Design review of the part built by this model. Coordinates are the model's own, in mm. A direction names the side the tool comes from. Give positions to 0.01 mm unless a question says otherwise; leave off trailing zeros. Write each loop counter-clockwise with the first axis right and the second up, starting at its lowest first coordinate (ties: lowest second). Pieces come first, ordered by that corner, then holes. Notation, with made-up numbers: M 42.25,86 L 90.25,86 A35 ccw 90.25,124 Z; hole C -23,48.5 d10. An arc over 180 degrees is marked long. Answer in a Markdown table with one row per item.
```python
from build123d import *

# Parameters (mm, degrees)
PAD012_DEPTH    = 1
SKETCH027_W     = 2.8
SKETCH027_H     = 5
PAD013_DEPTH    = 3.1
SKETCH028_W     = 14.36185
SKETCH028_H     = 25.638802
PAD014_DEPTH    = 0.5
SKETCH029_W     = 4.6
SKETCH029_H     = 6.5
PAD015_DEPTH    = 1
SKETCH030_W     = 4.91
SKETCH030_H     = 1.11
PAD016_DEPTH    = 2.9
CHAMFER003_SIZE = 0.8


with BuildPart() as part:
    # Sketch026 → Pad012 (new body)
    with BuildSketch(Plane.XY.offset(-6.5)):
        Polygon((-24.727272, 35.025402), (16.242728, 35.025402), (16.242728, -17.564598), (-24.727272, -17.564598), (-24.727272, -10.26), (-22.927272, -10.26), (-22.927272, -5.76), (-24.727272, -5.76), (-24.727272, 22.57), (-22.927272, 22.57), (-22.927272, 27.07), (-24.727272, 27.07), align=None)
    extrude(amount=PAD012_DEPTH)

    # Sketch027 (on Face14 of Pad012) → Pad013 (join)
    with BuildSketch(Plane.XY.offset(-5.5)):
        with Locations((-21.4, -8.066671)):
            Rectangle(SKETCH027_W, SKETCH027_H)
        with Locations((-21.4, 24.933329)):
            Rectangle(SKETCH027_W, SKETCH027_H)
    extrude(amount=PAD013_DEPTH)

    # Sketch028 (on Face5 of Pad013) → Pad014 (join)
    with BuildSketch(Plane.XY.offset(-5.5)):
        Polygon((15.9, -11.144853), (-22.75, -11.144853), (-22.75, -4.144854), (-16.362574, -4.144854), (-16.362574, 21.495147), (-22.75, 21.495147), (-22.75, 28.495147), (15.9, 28.495147), (15.9, 21.495148), (9.999276, 21.495148), (9.999276, -4.144854), (15.9, -4.144854), align=None)
        with Locations((-3.181649, 8.674547)):
            Rectangle(SKETCH028_W, SKETCH028_H, mode=Mode.SUBTRACT)
    extrude(amount=PAD014_DEPTH)

    # Sketch029 (on Face35 of Pad014) → Pad015 (join)
    with BuildSketch(Plane.XY.offset(-5)):
        with Locations((16.17, 24.951215)):
            Rectangle(SKETCH029_W, SKETCH029_H)
        with Locations((16.17, -7.83)):
            Rectangle(SKETCH029_W, SKETCH029_H)
    extrude(amount=PAD015_DEPTH)

    # Sketch030 (on Face34 of Pad015) → Pad016 (join)
    with BuildSketch(Plane(origin=(-22.8, 0, 0), x_dir=(0, -1, 0), z_dir=(-1, 0, 0))):
        with Locations((-24.925, -3.103053)):
            Rectangle(SKETCH030_W, SKETCH030_H)
        with Locations((8.065, -3.103053)):
            Rectangle(SKETCH030_W, SKETCH030_H)
    extrude(amount=PAD016_DEPTH)

    # Chamfer003
    chamfer003_edges = [part.edges().sort_by_distance(p)[0] for p in [
        (-25.7, 24.925, -2.548053),
        (-25.7, -8.065, -2.548053),
        (-20, 24.933329, -2.4),
        (-20, -8.066671, -2.4),
        (-20, 24.933329, -5),
        (-20, -8.066671, -5),
        (-22.8, -8.065, -3.658053),
        (-22.8, 24.925, -3.658053),
    ]]
    chamfer(chamfer003_edges, length=CHAMFER003_SIZE)


with BuildPart() as part_1:
    # Body005 placement: moved
    add(part.part.moved(Location((1, 2, -1.7))))


solid = part_1.part
```
1) For faces 4 (the face through (17, -6, -5.7)), 5 (the face through (-23, -8.52, -5)), 6 (the face through (-2, 11, -7.2)), list the 3-axis set-ups (+Z, -Z, +X, -X, +Y, -Y) from which the entire face can be reached by the end or side of a thin tool; tool diameter is ignored.
Geometry says:
| item | result |
|---|---|
| face 4 | +Z, +X, +Y, -Y |
| face 5 | +Z, -X, -Y |
| face 6 | +Z |
2) The part is to be moulded in two halves that separate along Z. For faces 1 (the face through (-21.8, -6.08, -6.35)), 2 (the face through (-21, -6, -4.1)), 3 (the face through (-23, 29.38, -5)), say which applies: released by +Z, released by -Z, zero draft, split by the parting line, or undercut.
Geometry says:
| item | result |
|---|---|
| face 1 | undercut |
| face 2 | released by +Z |
| face 3 | zero draft |
3) To check wall thickness, follow probe 1 along Y at (x, z) = (-7.5, -6.9); probe 2 along Z at (x, y) = (10, 14.5); probe 3 along X at (y, z) = (27.5, -6.8). State the ranges of each line that lie inside material, in increasing order. Write a range as [from, to].
Geometry says:
| item | result |
|---|---|
| probe 1 | [-9.14, -2.14], [23.49, 30.5] |
| probe 2 | [-8.2, -6.7] |
| probe 3 | [-21.8, 16.9] |
4) Insertion check: P1, Ø19.5, axis at x = 3, y = 20, coming from the +Z side; P2, Ø1.5, axis at x = -23.5, z = -5, coming from the +Y side; P3, Ø2.5, axis at x = -22.5, y = -7, coming from the +Z side; P4, Ø1, axis at x = -0.5, z = -6.5, coming from the -Y side. Each pin has a flat end and moves straight along its axis. Give the tip position at first contact, or say it passes through.
Geometry says:
| item | result |
|---|---|
| P1 | z = -6.7 |
| P2 | y = 29.38 |
| P3 | z = -4.1 |
| P4 | y = -9.14 |
5) Add section A-A (y = -7.5). Write out the cut boundary in (x, z).
Geometry says:
| item | result |
|---|---|
| outline | M -24.7,-5.36 L -22.6,-5.36 L -21.8,-6.16 L -21.8,-7.2 L -21.93,-7.2 L -21.93,-8.2 L 17.24,-8.2 L 17.24,-7.2 L 16.9,-7.2 L 16.9,-6.7 L 19.47,-6.7 L 19.47,-5.7 L 14.87,-5.7 L 14.87,-6.7 L -18.2,-6.7 L -19,-5.9 L -19,-4.9 L -19.8,-4.1 L -21.8,-4.1 L -21.8,-4.25 L -23.9,-4.25 L -24.7,-5.05 Z |
6) Add section C-C (y = 17.5). Write out the cut boundary in (x, z).
Geometry says:
| item | result |
|---|---|
| outline | M -23.73,-8.2 L 17.24,-8.2 L 17.24,-7.2 L 11,-7.2 L 11,-6.7 L 5,-6.7 L 5,-7.2 L -9.36,-7.2 L -9.36,-6.7 L -15.36,-6.7 L -15.36,-7.2 L -23.73,-7.2 Z |
7) Add section B-B (x = -6). Write out the cut boundary in (y, z).
Geometry says:
| item | result |
|---|---|
| outline | M -15.56,-8.2 L 37.03,-8.2 L 37.03,-7.2 L 30.5,-7.2 L 30.5,-6.7 L 23.49,-6.7 L 23.49,-7.2 L -2.14,-7.2 L -2.14,-6.7 L -9.14,-6.7 L -9.14,-7.2 L -15.56,-7.2 Z |
